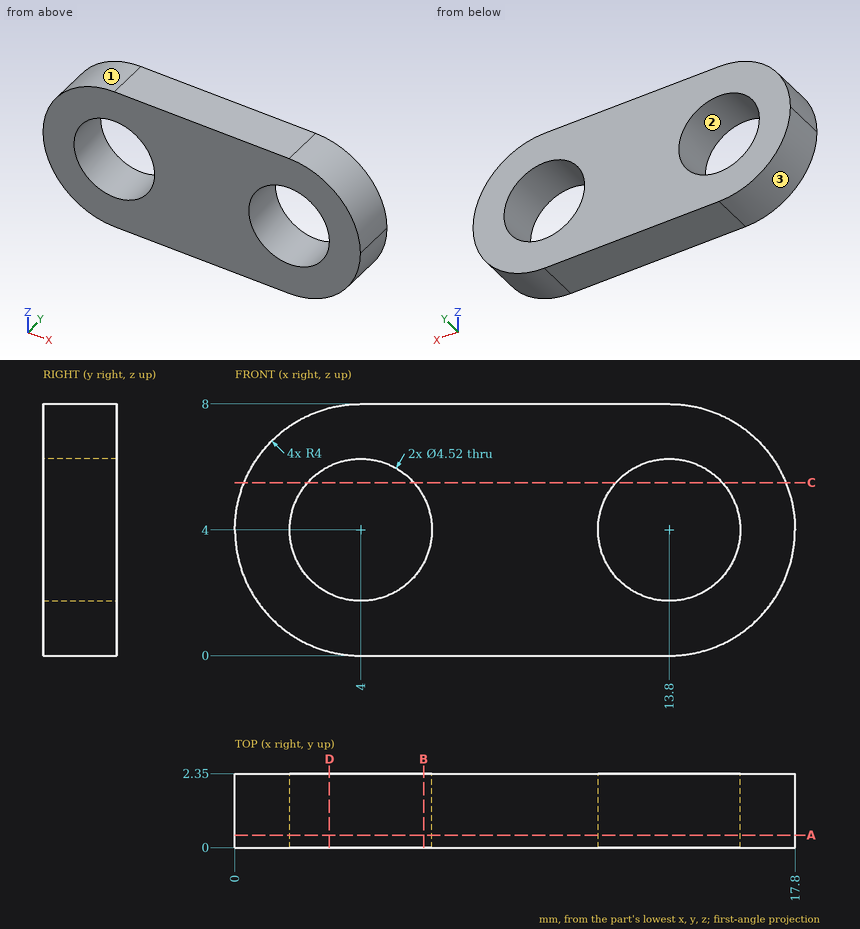
Job drawing, mm, ordinate dimensions from the low corner. One solid piece. Coordinates: 2 decimals unless noted, no trailing zeros. Write each loop counter-clockwise with the first axis right and the second up, starting at its lowest first coordinate (ties: lowest second). Pieces come first, ordered by that corner, then holes.
Item 1: Slice it at C-C (z = 5.5). Write the cut outline in (x, y).
Item 2: Probe line 1 (X direction, y = 1.85, z = 4); line 2 (X direction, y = 0.2, z = 5.25); line 3 (Z direction, x = 13.75, y = 0.4). List the from-to ranges inside material, lowest first.
Item 3: Slice it at D-D (x = 3). Write the cut outline in (y, z).
Item 4: Mould opens along Z. For the marked faces 1, 2 and 3 say: released by +Z, released by -Z, zero draft, split by the parting line, or undercut.
Item 5: Pin check, flat tip, straight feed: pin 1 (1 mm diameter, centred on y = 0.5, z = 5, fed in from -X). Stop position of the tip, or through.
Item 6: Slice it at A-A (y = 0.4). Count the separate pieces of the cut face and the enclosed holes in it, and give its area (3 significant figures).
Item 7: Slice it at B-B (x = 6). Write the cut outline in (y, z).
Results found:
1. outline: (0.29, 0) - (2.31, 0) - (2.31, 2.35) - (0.29, 2.35) - close; (5.69, 0) - (12.11, 0) - (12.11, 2.35) - (5.69, 2.35) - close; (15.49, 0) - (17.51, 0) - (17.51, 2.35) - (15.49, 2.35) - close
2. line 1: x = 0 to 1.74, 6.26 to 11.54, 16.06 to 17.8
2. line 2: x = 0.2 to 2.12, 5.88 to 11.92, 15.68 to 17.6
2. line 3: z = 0 to 1.74, 6.26 to 8
3. outline: (0, 0.13) - (2.35, 0.13) - (2.35, 1.97) - (0, 1.97) - close; (0, 6.03) - (2.35, 6.03) - (2.35, 7.87) - (0, 7.87) - close
4. face 1: released by +Z
4. face 2: undercut
4. face 3: released by -Z
5. pin 1: stops at x = 0.03
6. separate pieces: 1
6. enclosed holes: 2
6. area: 96.6 mm2
7. outline: (0, 0) - (2.35, 0) - (2.35, 2.95) - (0, 2.95) - close; (0, 5.05) - (2.35, 5.05) - (2.35, 8) - (0, 8) - close
